```python
from build123d import *

# Parameters (mm, degrees)
F3_DEPTH        = 2.9
F5_DEPTH        = 20
F7_DEPTH        = 2.9
F7_COPIES_COUNT = 6


# Not quite as in the source:
# - a pattern or mirror of a feature is missing from the dataset's text; its kind, count and spacing are read off the source's solid


with BuildPart() as f1:
    # F0 (on Front) → F1 (revolve)
    with BuildSketch(Plane.XZ):
        Polygon((1.6, 16.3), (3.5, 16.3), (3.5, 19.3), (-4.5, 19.3), (-4.5, 0), (0, 0), (0, 13.3), align=None)
    revolve(axis=Axis((15.3209697455, 0, 0), (1, 0, 0)))

    # F2 (on face) → F3 (join)
    with BuildSketch(Plane.YZ):
        Polygon((-2.1073284825, 3.65), (-4.2146569651, 0), (-2.1073284825, -3.65), (2.1073284825, -3.65), (4.2146569651, 0), (2.1073284825, 3.65), align=None)
    extrude(amount=F3_DEPTH)

    # F4 (on face) → F5 (join)
    with BuildSketch(Plane(origin=(-4.5, 0, 0), x_dir=(0, -1, 0), z_dir=(-1, 0, 0))):
        Polygon((0, 18.4752086141), (-16, 9.237604307), (-16, -9.237604307), (0, -18.4752086141), (16, -9.237604307), (16, 9.237604307), align=None)
    extrude(amount=F5_DEPTH)

    # F6 (on face) → F7 (join)
    with BuildSketch(Plane.YZ):
        with BuildLine():
            Line((1.45, 15), (-1.45, 15))
            Line((-1.45, 15), (-1.45, 12.55))
            ThreePointArc((-1.45, 12.55), (0, 11.1), (1.45, 12.55))
            Line((1.45, 12.55), (1.45, 15))
        make_face()
    f7 = extrude(amount=F7_DEPTH)

    # F7_copies: F7 ×6 about axis
    f7_copies_axis = Axis((0, 0, 0), (1, 0, 0))
    for i in range(1, F7_COPIES_COUNT):
        add(f7.rotate(f7_copies_axis, i * 360 / F7_COPIES_COUNT))


solid = f1.part
```
Verification items for the finished model (mm, model axes). A direction names the side the tool comes from. Round coordinates to 2 decimals unless told otherwise and drop trailing zeros. Write each loop counter-clockwise with the first axis right and the second up, starting at its lowest first coordinate (ties: lowest second). Pieces come first, ordered by that corner, then holes. Notation, with made-up numbers: (51, -27.75) - (87, -27.75) arc R37 ccw to (87, 9.25) - close; hole circle Ø2 at (-6.5, 8). An arc over 180 degrees is marked (long way). Answer as a JSON object with one key per item and string values. Group by question number.
Q1. Mould release check, pull along Z, two halves, no side actions. Record for faces 5 (the cylindrical face through (-0.556, -5.797, 18.409)), 6 (the flat face through (1.4, 12.6, 5.6)), 7 (the cylindrical face through (2.563, 9.918, -12.935)), 8 (the flat face through (3.5, 4, 16)): released by +Z, released by -Z, zero draft, split by the parting line, or undercut.
Q2. Section check A-A, the plane x = -21.75. Enter the section's corners in (y, z).
Q3. Tool access check on faces 1 (the flat face through (-4.5, 10, 13)), 2 (the flat face through (1.43, -3.146, 1.851)), 3 (the flat face through (-14, 16, 0)), 4 (the flat face through (-14.36, -7.89, -13.92)). Record the directions out of +Z, -Z, +X, -X, +Y, -Y that give a thin tool (end or side, any length) a straight path to the whole face; none if there is none.
Q4. Go/stop test with flat-tipped pins: pin 1 Ø1.5 at (x, z) = (-3, -11.5) entering from +Y; pin 2 Ø1.5 at (y, z) = (0.5, -13) entering from +X; pin 3 Ø4 at (x, y) = (-14, 10) entering from +Z. Record where each tip stops, or that it passes through.
Q5. Thickness scan on line 1 (Y direction, x = 2, z = 0); line 2 (Z direction, x = 2.4, y = 0); line 3 (Z direction, x = 1.5, y = -1.5). Record the ranges inside material, lowest first.
Found:
{
 "1": {"face 5": "split by the parting line", "face 6": "undercut", "face 7": "undercut", "face 8": "zero draft"},
 "2": {"outline": "(-16, -9.24) - (0, -18.48) - (16, -9.24) - (16, 9.24) - (0, 18.48) - (-16, 9.24) - close"},
 "3": {"face 1": "-X", "face 2": "+X", "face 3": "+Z, -Z, -X, +Y", "face 4": "-Z, -X, -Y"},
 "4": {"pin 1": "stops at y = 16.03", "pin 2": "stops at x = 2.9", "pin 3": "stops at z = 13.86"},
 "5": {"line 1": "y = -19.3 to -16.3, -4.21 to 4.21, 16.3 to 19.3", "line 2": "z = -19.3 to -16.3, -15 to -11.1, -3.65 to 3.65, 11.1 to 15, 16.3 to 19.3", "line 3": "z = -19.24 to -16.04, -3.65 to 3.65, 16.04 to 19.24"}
}
